Autodesk Inventor part; units mm, degrees
ref_plane "YZ Plane" through (0, 0, 0) normal (1, 0, 0) x (0, 1, 0)
ref_plane "XZ Plane" through (0, 0, 0) normal (0, 1, 0) x (-1, 0, 0)
ref_plane "XY Plane" through (0, 0, 0) normal (0, 0, 1) x (1, 0, 0)
sketch "Sketch1" plane through (0, 0, 0) normal (0, 0, 1) x (1, 0, 0)
  line L0 (0, 7.3323) -> (6.35, 3.6662)
  line L1 (6.35, 3.6662) -> (6.35, -3.6662)
  line L2 (6.35, -3.6662) -> (0, -7.3323)
  line L3 (0, -7.3323) -> (-6.35, -3.6662)
  line L4 (-6.35, -3.6662) -> (-6.35, 3.6662)
  line L5 (-6.35, 3.6662) -> (0, 7.3323)
  point P0 (0, 0)
  point P1 (0, 0)
  dimension "d0" = 12.7
extrude "Extrusion1" add sketch "Sketch1" along normal blind 152.4
sketch "Sketch2" plane through (0, 0, 152.4) normal (0, 0, 1) x (1, 0, 0)
  circle A0 centre (0, 0) radius 9.525
  line L0 (-6.35, 3.6662) -> (-6.35, -3.6662)
  line L1 (6.35, 3.6662) -> (0, 7.3323)
  line L2 (0, 7.3323) -> (-6.35, 3.6662)
  line L3 (-6.35, 3.6662) -> (-6.35, -3.6662)
  line L4 (-6.35, -3.6662) -> (0, -7.3323)
  line L5 (0, -7.3323) -> (6.35, -3.6662)
  line L6 (6.35, -3.6662) -> (6.35, 3.6662)
  line L7 (-6.35, 3.6662) -> (-6.35, 7.0995)
  line L8 (-6.35, -3.6662) -> (-6.35, -7.0995)
  point P0 (-6.35, -3.6662)
  dimension "d3" = 19.05
extrude "Extrusion2" add sketch "Sketch2" along normal blind 2.54 contours A0 L8 L4 L5 L6 L1 L2 L7 | L2 L1 L6 L5 L4 L0
properties part number "_3DPrint"
Design review of the part built by this model. Coordinates are the model's own, in mm. A direction names the side the tool comes from. Round coordinates to 2 decimals unless told otherwise and drop trailing zeros. Write each loop counter-clockwise with the first axis right and the second up, starting at its lowest first coordinate (ties: lowest second). Pieces come first, ordered by that corner, then holes.
Item 1: For pin 1 Ø6 at (y, z) = (-0.5, 98.5) entering from +X; pin 2 Ø5 at (x, z) = (-4.5, 25) entering from -Y; pin 3 Ø3 at (x, y) = (-0.5, 7.5) entering from -Z; pin 4 Ø1 at (x, z) = (-3.5, 45) entering from +Y, all flat-tipped, find the tip position at first contact; note any pin that passes through.
Item 2: For faces 1 (the flat face through (7, 0, 152.4)), 2 (the flat face through (-3.219, 5.474, 75.133)), 3 (the flat face through (6.35, 0, 75)), 4 (the flat face through (-3.131, -5.525, 75.133)), 5 (the flat face through (3.131, 5.525, 75.133)), list the 3-axis set-ups (+Z, -Z, +X, -X, +Y, -Y) from which the entire face can be reached by the end or side of a thin tool; tool diameter is ignored.
Item 3: Wall thickness on L1, parallel to Z at x = 3.5, y = 7.75; L2, parallel to X at y = 2.5, z = 22.5; L3, parallel to Y at x = 0, z = 132: over which ranges is each line inside the solid? List them lowest first.
Item 4: Consider section A-A on y = 0. Give the boundary of the cut face in (x, z) (3 decimals).
Item 5: Consider section B-B on z = 15.5. Give the boundary of the cut face in (x, y).
Item 6: Consider section C-C on x = 2. Give the boundary of the cut face in (y, z).
Check values:
1. pin 1: stops at x = 6.35
1. pin 2: stops at y = -6.18
1. pin 3: stops at z = 0
1. pin 4: stops at y = 5.6
2. face 1: -Z
2. face 2: -Z, -X, +Y
2. face 3: -Z, +X, +Y, -Y
2. face 4: -Z, -X, -Y
2. face 5: -Z, +X, +Y
3. L1: z = 152.4 to 154.94
3. L2: x = -6.35 to 6.35
3. L3: y = -7.33 to 7.33
4. outline: (-6.35, 0) - (6.35, 0) - (6.35, 152.4) - (9.525, 152.4) - (9.525, 154.94) - (-6.35, 154.94) - close
5. outline: (-6.35, -3.67) - (0, -7.33) - (6.35, -3.67) - (6.35, 3.67) - (0, 7.33) - (-6.35, 3.67) - close
6. outline: (-9.31, 152.4) - (-6.18, 152.4) - (-6.18, 0) - (6.18, 0) - (6.18, 152.4) - (9.31, 152.4) - (9.31, 154.94) - (-9.31, 154.94) - close
